The figure shows three views and two pictorial views of one solid part (mm, origin at its lowest corner). Answer the questions. A direction names the side the tool comes from. Give positions to 0.01 mm unless a question says otherwise; leave off trailing zeros. Loops run counter-clockwise (first coordinate to the right, second up) from the corner with the lowest first, then second, coordinate; pieces in that order, holes last. Notation, with made-up numbers: (36, 53.5) - (88, 53.5) arc R33 cw to (88, 91.5) - close; hole circle Ø7 at (71, -30.75). An arc over 180 degrees is marked (long way). Write each question's results on one line, items separated by ' | '.
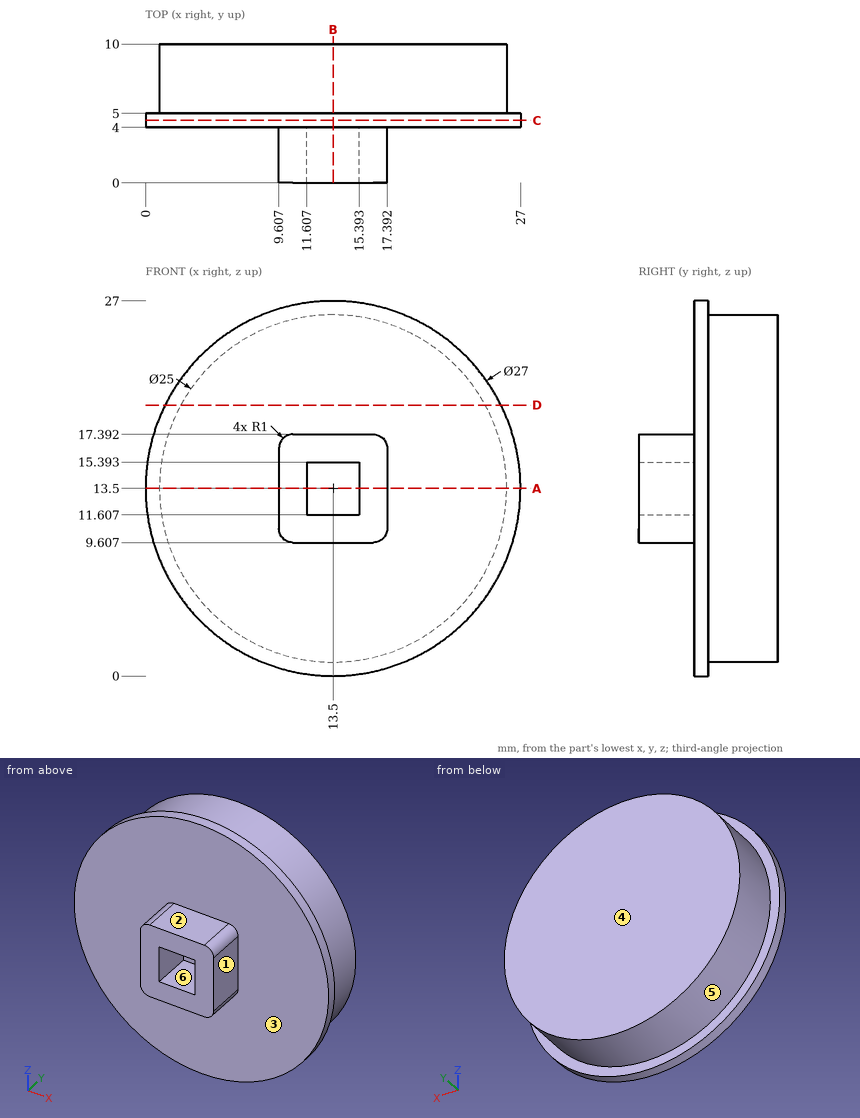
Item 1: A cutting plane is placed at A-A, the plane z = 13.5. Determine the outline of the cut face in (x, y).
Values found:
outline: (0, 4) - (9.61, 4) - (9.61, 0) - (11.61, 0) - (11.61, 4) - (15.39, 4) - (15.39, 0) - (17.39, 0) - (17.39, 4) - (27, 4) - (27, 5) - (26, 5) - (26, 10) - (1, 10) - (1, 5) - (0, 5) - close
Item 2: For a pull along Z with two mould halves and no side action, classify the marked faces 4, 5 and 6 as released by +Z, released by -Z, zero draft, split by the parting line, or undercut.
Values found:
face 4: zero draft | face 5: split by the parting line | face 6: undercut
Item 3: For the marked faces 1, 2 and 3, determine the directions among +Z, -Z, +X, -X, +Y, -Y from which every point of the face is accessible in a straight line to the end or side of a thin tool.
Values found:
face 1: +Z, -Z, +X, -Y | face 2: +Z, +X, -X, -Y | face 3: -Y
Item 4: A cutting plane is placed at B-B, the plane x = 13.5. Determine the outline of the cut face in (y, z), plus the area to 3 significant figures.
Values found:
outline: (0, 9.61) - (4, 9.61) - (4, 0) - (5, 0) - (5, 1) - (10, 1) - (10, 26) - (5, 26) - (5, 27) - (4, 27) - (4, 17.39) - (0, 17.39) - (0, 15.39) - (4, 15.39) - (4, 11.61) - (0, 11.61) - close | area: 168 mm²
Item 5: Find the intervals of material crossed by line 1 along Y through (x, z) = (1, 10); line 2 along Z through (x, y) = (15.25, 2.25); line 3 along Y through (x, z) = (23.5, 19.25), in increasing order. Write a range as [from, to].
Values found:
line 1: y = [4, 5] | line 2: z = [9.61, 11.61], [15.39, 17.39] | line 3: y = [4, 10]
Item 6: A cutting plane is placed at C-C, the plane y = 4.5. Determine the outline of the cut face in (x, z).
Values found:
outline: circle Ø27 at (13.5, 13.5)
Item 7: Flat-ended cylindrical pins translate along their axes: P1, Ø6, axis at x = 5.5, z = 13.5, coming from the -Y side; P2, Ø1.1, axis at y = 2, z = 14, coming from the -X side; P3, Ø1.1, axis at x = 13, y = 2, coming from the -Z side. Find the tip coordinate at first contact, or state that the pin passes through.
Values found:
P1: stops at y = 4 | P2: stops at x = 9.61 | P3: stops at z = 9.61
Item 8: A cutting plane is placed at D-D, the plane z = 19.5. Determine the outline of the cut face in (x, y) (1 decimal), plus the area to 3 significant figures.
Values found:
outline: (1.4, 4) - (25.6, 4) - (25.6, 5) - (24.5, 5) - (24.5, 10) - (2.5, 10) - (2.5, 5) - (1.4, 5) - close | area: 134 mm²
